Verification items for this drawing (mm, ordinates from the low corner). Give positions to 0.01 mm unless a question says otherwise; leave off trailing zeros. Order: outer loops, then holes, each group sorted by start corner. A loop starts at its lowest first (then second) coordinate and runs counter-clockwise, first axis right, second up. Notation, with made-up numbers: M 21,53 L 68,53 A24 cw 68,65 Z; hole C 3.25,-17 d2. An arc over 180 degrees is marked long. Answer as a JSON object with one key per item and string values.
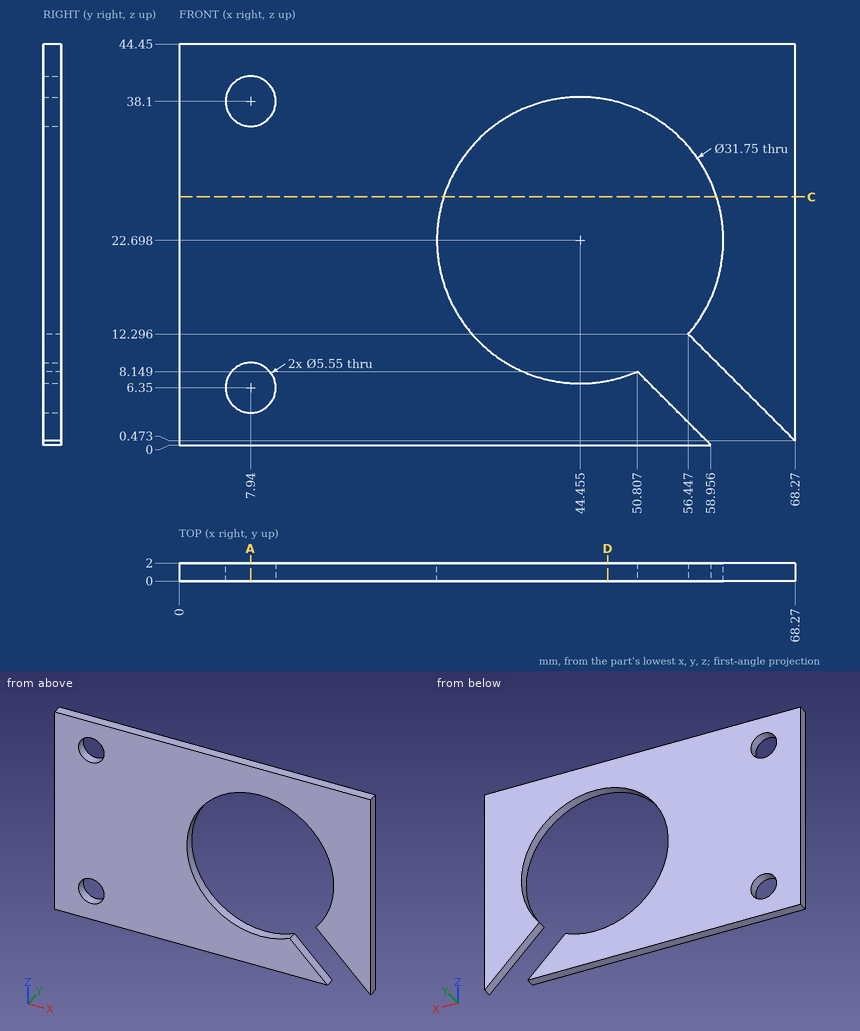
Q1. Material ranges on L1, parallel to X at y = 0.7, z = 4 (1 decimal); L2, parallel to Z at x = 10, y = 0.75; L3, parallel to Z at x = 44.5, y = 0.25, recorded low to high.
Resolved:
{"L1": "x = 0 to 6.5, 9.4 to 55, 64.7 to 68.3", "L2": "z = 0 to 4.49, 8.21 to 36.24, 39.96 to 44.45", "L3": "z = 0 to 6.82, 38.57 to 44.45"}
Q2. Section check D-D on x = 47.5. Record the cut outline in (y, z).
Resolved:
{"outline": "M 0,0 L 2,0 L 2,7.12 L 0,7.12 Z; M 0,38.28 L 2,38.28 L 2,44.45 L 0,44.45 Z"}
Q3. Section check A-A on x = 7.94. Count the separate pieces of the cut face and the enclosed holes in it.
Resolved:
{"separate pieces": "3", "enclosed holes": "0"}
Q4. Section check C-C on z = 27.5. Record the cut outline in (x, y).
Resolved:
{"outline": "M 0,0 L 29.32,0 L 29.32,2 L 0,2 Z; M 59.59,0 L 68.27,0 L 68.27,2 L 59.59,2 Z"}
